from build123d import *

# Parameters (mm, degrees)
SKETCH_1_R               = 75
SKETCH_1_R_2             = 2.65
EXTRUDE_1_DEPTH          = 10
SKETCH_2_R               = 65
SKETCH_2_R_2             = 52.5
EXTRUDE_2_DEPTH          = 2
SKETCH_3_R               = 65
SKETCH_3_R_2             = 57.5
EXTRUDE_3_DEPTH          = 13
EXTRUDE_START            = -5
SKETCH_4_R               = 2.15
EXTRUDE_4_DEPTH          = 5
PATTERN_CIRCULAR_1_COUNT = 6
FILLET_1_R               = 3
CUT_EXTRUDE_START        = -80
SKETCH_6_R               = 52.5
CUT_EXTRUDE_1_DEPTH      = 80


with BuildPart() as part:
    # 草图1 → 凸台-拉伸1 (new body)
    with BuildSketch(Plane(origin=(0, 0, 0), x_dir=(1, 0, 0), z_dir=(0, 1, 0))):
        with Locations(Location((0, 0, 0), (0, 0, 270))):
            Circle(SKETCH_1_R)
        with Locations(Location((0, 70, 0), (0, 0, 270))):
            Circle(SKETCH_1_R_2, mode=Mode.SUBTRACT)
        with Locations(Location((60.621778265, 35, 0), (0, 0, 270))):
            Circle(SKETCH_1_R_2, mode=Mode.SUBTRACT)
        with Locations(Location((60.621778265, -35, 0), (0, 0, 270))):
            Circle(SKETCH_1_R_2, mode=Mode.SUBTRACT)
        with Locations(Location((0, -70, 0), (0, 0, 270))):
            Circle(SKETCH_1_R_2, mode=Mode.SUBTRACT)
        with Locations(Location((-60.621778265, -35, 0), (0, 0, 270))):
            Circle(SKETCH_1_R_2, mode=Mode.SUBTRACT)
        with Locations(Location((-60.621778265, 35, 0), (0, 0, 270))):
            Circle(SKETCH_1_R_2, mode=Mode.SUBTRACT)
    extrude(amount=EXTRUDE_1_DEPTH)

    # 草图2 → 凸台-拉伸2 (add)
    with BuildSketch(Plane(origin=(0, 10, 0), x_dir=(1, 0, 0), z_dir=(0, 1, 0))):
        with Locations(Location((0, 0, 0), (0, 0, 270))):
            Circle(SKETCH_2_R)
        with Locations(Location((0, 0, 0), (0, 0, 270))):
            Circle(SKETCH_2_R_2, mode=Mode.SUBTRACT)
    extrude(amount=EXTRUDE_2_DEPTH)

    # 草图3 → 凸台-拉伸3 (add)
    with BuildSketch(Plane(origin=(0, 12, 0), x_dir=(1, 0, 0), z_dir=(0, 1, 0))):
        with Locations(Location((0, 0, 0), (0, 0, 270))):
            Circle(SKETCH_3_R)
        with Locations(Location((0, 0, 0), (0, 0, 90))):
            Circle(SKETCH_3_R_2, mode=Mode.SUBTRACT)
    extrude(amount=EXTRUDE_3_DEPTH)

    # 草图4 → 凸台-拉伸4 (add)
    with BuildSketch(Plane(origin=(0, 25, 0), x_dir=(1, 0, 0), z_dir=(0, 1, 0)).offset(EXTRUDE_START)):
        with BuildLine():
            Line((-53.033008589, 53.033008589), (-45.961940777, 45.961940777))
            ThreePointArc((-45.961940777, 45.961940777), (-32.5, 56.291651246), (-16.823237932, 62.785178709))
            Line((-16.823237932, 62.785178709), (-19.411428383, 72.444436972))
            ThreePointArc((-19.411428383, 72.444436972), (-37.5, 64.951905284), (-53.033008589, 53.033008589))
        make_face()
        with Locations(Location((-35, 60.621778265, 0), (0, 0, 270))):
            Circle(SKETCH_4_R, mode=Mode.SUBTRACT)
    extrude_4 = extrude(amount=EXTRUDE_4_DEPTH)

    # 阵列(圆周)1: 凸台-拉伸4 ×6 about axis
    pattern_circular_1_axis = Axis((0, 0, 0), (0, 1, 0))
    for i in range(1, PATTERN_CIRCULAR_1_COUNT):
        add(extrude_4.rotate(pattern_circular_1_axis, i * 360 / PATTERN_CIRCULAR_1_COUNT))

    # 圆角1
    fillet_1_edges = [part.edges().sort_by_distance(p)[0] for p in [
        (62.785178709, 22.5, -16.823237932),
        (72.444436972, 22.5, -19.411428383),
        (72.444436972, 22.5, 19.411428383),
        (45.961940777, 22.5, -45.961940777),
        (16.823237932, 22.5, -62.785178709),
        (19.411428383, 22.5, -72.444436972),
        (53.033008589, 22.5, -53.033008589),
        (-16.823237932, 22.5, -62.785178709),
        (-45.961940777, 22.5, -45.961940777),
        (-53.033008589, 22.5, -53.033008589),
        (-19.411428383, 22.5, -72.444436972),
        (-62.785178709, 22.5, -16.823237932),
        (-62.785178709, 22.5, 16.823237932),
        (-72.444436972, 22.5, 19.411428383),
        (-72.444436972, 22.5, -19.411428383),
        (-45.961940777, 22.5, 45.961940777),
        (-16.823237932, 22.5, 62.785178709),
        (-19.411428383, 22.5, 72.444436972),
        (-53.033008589, 22.5, 53.033008589),
        (16.823237932, 22.5, 62.785178709),
        (45.961940777, 22.5, 45.961940777),
        (53.033008589, 22.5, 53.033008589),
        (19.411428383, 22.5, 72.444436972),
        (62.785178709, 22.5, 16.823237932),
    ]]
    fillet(fillet_1_edges, radius=FILLET_1_R)

    # 草图6 → 切除-拉伸1 (cut)
    with BuildSketch(Plane(origin=(0, 10, 0), x_dir=(1, 0, 0), z_dir=(0, 1, 0)).offset(CUT_EXTRUDE_START)):
        with Locations(Location((0, 0, 0), (0, 0, 270))):
            Circle(SKETCH_6_R)
    extrude(amount=CUT_EXTRUDE_1_DEPTH, mode=Mode.SUBTRACT)


solid = part.part
The model under review builds one solid part; all positions refer to its coordinate system, in mm. A direction names the side the tool comes from. Round coordinates to 2 decimals unless told otherwise and drop trailing zeros. Loops run counter-clockwise (first coordinate to the right, second up) from the corner with the lowest first, then second, coordinate; pieces in that order, holes last. Notation, with made-up numbers: M 44,-14 L 75,-14 A28 ccw 75,8 Z; hole C -6,38.25 d10. An arc over 180 degrees is marked long. Answer as CSV lines item,"result". Start each with the question number.
Item 1: Consider section D-D (z = 35). Write out the cut boundary in (x, y).
Item 2: Mouldability with a two-part tool opening along X and no side actions: class faces 1 (the face through (34, 20, -57)), 2 (the face through (18.093, 22.465, 67.526)), 3 (the face through (47.158, 22.535, -45.949)) as released by +X, released by -X, zero draft, split by the parting line, or undercut.
Item 3: Consider section A-A (x = 0). Write out the cut boundary in (y, z), then the cut area to 3 significant figures.
Item 4: Consider section C-C (y = 7). Write out the cut boundary in (x, z).
Item 5: For faces 4 (the face through (-20, 22.5, 71.3)), 5 (the face through (-34, 20, 57)), 6 (the face through (-47.158, 22.535, 45.949)), 7 (the face through (-63.372, 22.535, -17.865)), list the 3-axis set-ups (+Z, -Z, +X, -X, +Y, -Y) from which the entire face can be reached by the end or side of a thin tool; tool diameter is ignored.
Item 6: Wall thickness on line 1 (X direction, y = 13, z = -2); line 2 (X direction, y = 23, z = 0); line 3 (Y direction, x = -27, z = 65.5): over which ranges is each line inside the solid? List them lowest first. Write a range as [from, to].
Item 7: Insertion check: P1, Ø4, axis at x = -66.5, z = 0.5, coming from the -Y side; P2, Ø1.5, axis at x = -58, y = 13, coming from the +Z side; P3, Ø2.5, axis at x = 70, z = 0, coming from the +Y side; P4, Ø10, axis at y = 7.5, z = 35, coming from the -X side. Each pin has a flat end and moves straight along its axis. Give the tip position at first contact, or say it passes through.
Item 8: Consider section B-B (z = 4.5). Write out the cut boundary in (x, y).
Answer:
1,outline,"M -66.33,0 L -63.27,0 L -63.27,10 L -66.33,10 Z; M -57.97,0 L -39.13,0 L -39.13,12 L -45.62,12 L -45.62,25 L -54.77,25 L -54.77,10 L -57.97,10 Z; M 39.13,0 L 57.97,0 L 57.97,10 L 54.77,10 L 54.77,25 L 45.62,25 L 45.62,12 L 39.13,12 Z; M 63.27,0 L 66.33,0 L 66.33,10 L 63.27,10 Z"
2,face 1,"zero draft"
2,face 2,"undercut"
2,face 3,"released by +X"
3,outline,"M 0,-75 L 10,-75 L 10,-72.65 L 0,-72.65 Z; M 0,-67.35 L 10,-67.35 L 10,-65 L 25,-65 L 25,-57.5 L 12,-57.5 L 12,-52.5 L 0,-52.5 Z; M 0,52.5 L 12,52.5 L 12,57.5 L 25,57.5 L 25,65 L 10,65 L 10,67.35 L 0,67.35 Z; M 0,72.65 L 10,72.65 L 10,75 L 0,75 Z"
3,area,"589 mm^2"
4,outline,"C 0,0 d150; hole C -60.62,-35 d5.3; hole C -60.62,35 d5.3; hole C 0,0 d105; hole C 0,-70 d5.3; hole C 0,70 d5.3; hole C 60.62,-35 d5.3; hole C 60.62,35 d5.3"
5,face 4,"+Z, +Y"
5,face 5,"+Z, -X"
5,face 6,"-X, +Y"
5,face 7,"-Z, +Y"
6,line 1,"x = [-64.97, -57.47], [57.47, 64.97]"
6,line 2,"x = [-75, -72.15], [-67.85, -57.5], [57.5, 67.85], [72.15, 75]"
6,line 3,"y = [0, 10], [20, 25]"
7,P1,"stops at y = 0"
7,P2,"stops at z = 30.78"
7,P3,"stops at y = 10"
7,P4,"stops at x = -68.74"
8,outline,"M -74.86,0 L -52.31,0 L -52.31,12 L -57.32,12 L -57.32,25 L -74.86,25 L -74.86,20 L -64.84,20 L -64.84,10 L -74.86,10 Z; M 52.31,0 L 74.86,0 L 74.86,10 L 64.84,10 L 64.84,20 L 74.86,20 L 74.86,25 L 57.32,25 L 57.32,12 L 52.31,12 Z"
